Here's the drawing with two shaded views (mm, measured from the low corner). I have some questions. Round coordinates to 2 decimals unless told otherwise and drop trailing zeros. Write each loop counter-clockwise with the first axis right and the second up, starting at its lowest first coordinate (ties: lowest second). Pieces come first, ordered by that corner, then holes. Notation, with made-up numbers: (64, 53.25) -> (81, 53.25) arc R33 cw to (81, 87.25) -> close; hole circle Ø3 at (3.25, -23). An arc over 180 degrees is marked (long way). Use CSV: the item, a comma, the result in double quotes.
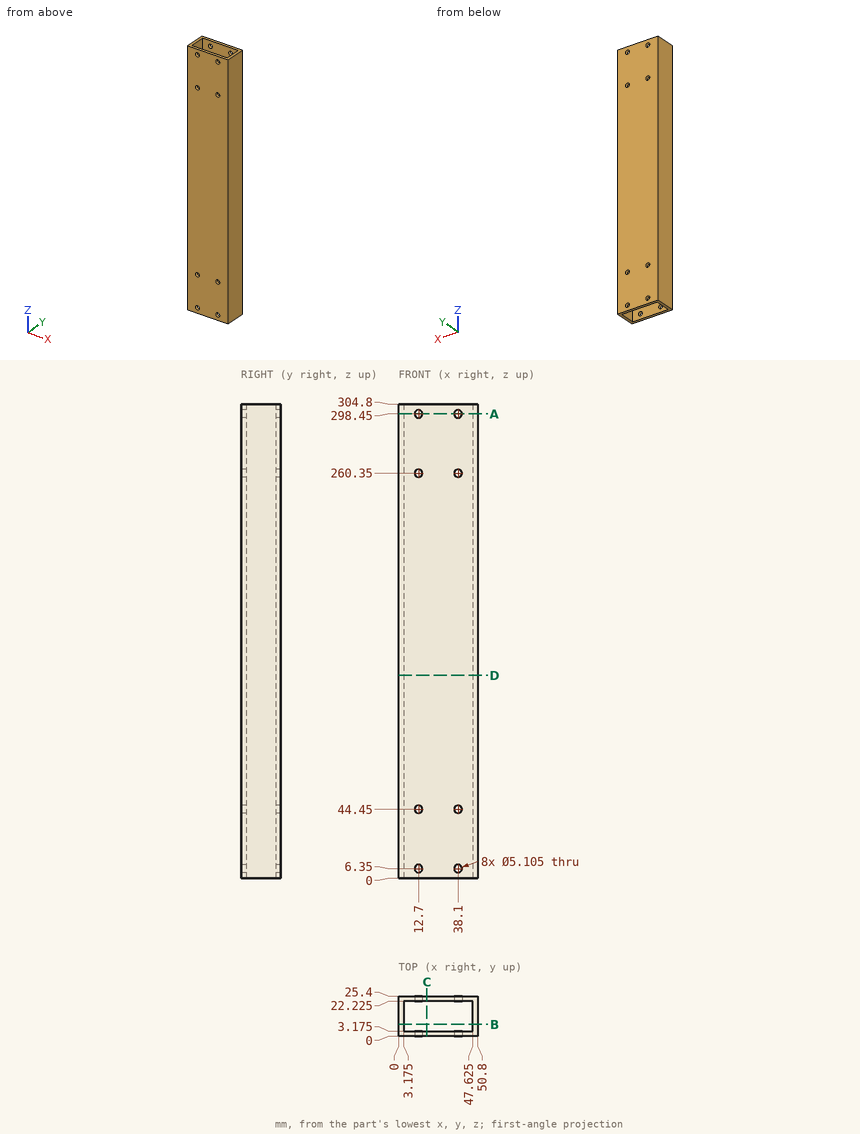
Q1. Suppose I cut it at A-A (z = 298.45). Write out the boundary of the cut face in (x, y) (1 decimal).
Resolved:
outline,"(0, 0) -> (10.1, 0) -> (10.1, 3.2) -> (3.2, 3.2) -> (3.2, 22.2) -> (10.1, 22.2) -> (10.1, 25.4) -> (0, 25.4) -> close; (15.3, 0) -> (35.5, 0) -> (35.5, 3.2) -> (15.3, 3.2) -> close; (15.3, 22.2) -> (35.5, 22.2) -> (35.5, 25.4) -> (15.3, 25.4) -> close; (40.7, 0) -> (50.8, 0) -> (50.8, 25.4) -> (40.7, 25.4) -> (40.7, 22.2) -> (47.6, 22.2) -> (47.6, 3.2) -> (40.7, 3.2) -> close"
Q2. Suppose I cut it at B-B (y = 7.5). Write out the boundary of the cut face in (x, z) (1 decimal).
Resolved:
outline,"(0, 0) -> (3.2, 0) -> (3.2, 304.8) -> (0, 304.8) -> close; (47.6, 0) -> (50.8, 0) -> (50.8, 304.8) -> (47.6, 304.8) -> close"
Q3. Suppose I cut it at D-D (z = 130.5). Write out the boundary of the cut face in (x, y) (1 decimal).
Resolved:
outline,"(0, 0) -> (50.8, 0) -> (50.8, 25.4) -> (0, 25.4) -> close; hole (3.2, 3.2) -> (47.6, 3.2) -> (47.6, 22.2) -> (3.2, 22.2) -> close"
Q4. Please list where these lines run through material, in increasing order: probe 1 along Z at (x, y) = (38.1, 1.35); probe 2 along X at (y, z) = (2.4, 260.35); probe 3 along Y at (x, z) = (32, 231) (1 decimal).
Resolved:
probe 1,"z = 0 to 3.8, 8.9 to 41.9, 47 to 257.8, 262.9 to 295.9, 301 to 304.8"
probe 2,"x = 0 to 10.15, 15.25 to 35.55, 40.65 to 50.8"
probe 3,"y = 0 to 3.2, 22.2 to 25.4"
Q5. Suppose I cut it at C-C (x = 18). Write out the boundary of the cut face in (y, z) (1 decimal).
Resolved:
outline,"(0, 0) -> (3.2, 0) -> (3.2, 304.8) -> (0, 304.8) -> close; (22.2, 0) -> (25.4, 0) -> (25.4, 304.8) -> (22.2, 304.8) -> close"
Q6. Will this pin go through, and if not, where does the flat tip stop? P1, Ø8, axis at x = 16, y = 15.5, coming from the -Z side.
Resolved:
P1,"passes through"
